Autodesk Inventor part; units mm, degrees
ref_plane "YZ Plane" through (0, 0, 0) normal (1, 0, 0) x (0, 1, 0)
ref_plane "XZ Plane" through (0, 0, 0) normal (0, 1, 0) x (-1, 0, 0)
ref_plane "XY Plane" through (0, 0, 0) normal (0, 0, 1) x (1, 0, 0)
sketch "Sketch1" plane through (0, 0, 0) normal (0, 0, 1) x (1, 0, 0)
  line L0 (-15.7, 12.7) -> (-12.7, 12.7)
  line L1 (-12.7, 12.7) -> (-12.7, -9.7)
  line L2 (-12.7, -9.7) -> (12.7, -9.7)
  line L3 (12.7, -9.7) -> (12.7, 12.7)
  line L4 (12.7, 12.7) -> (15.7, 12.7)
  line L5 (15.7, 12.7) -> (15.7, -12.7)
  line L6 (15.7, -12.7) -> (-15.7, -12.7)
  line L7 (-15.7, -12.7) -> (-15.7, 12.7)
  point P0 (0, 0)
  dimension "d0" = 3
  dimension "d2" = 3
  dimension "d3" = 25.4
  dimension "d4" = 31.4
  dimension "d5" = 15.7
  dimension "d7" = 12.7
  dimension "d8" = 3
extrude "Extrusion1" add sketch "Sketch1" against normal blind 660.4
sketch "Sketch5" plane through (15.7, -12.7, 0) normal (1, 0, 0) x (0, 0, -1)
  circle A0 centre (16, 12.7) radius 3.175
  circle A1 centre (644.4, 12.7) radius 3.175
  line L0 (0, 25.4) -> (0, 0)
  line L1 (660.4, 25.4) -> (660.4, 0)
  line L2 (0, 25.4) -> (660.4, 25.4)
  point P0 (0, 12.7)
  dimension "d56" = 6.35
  dimension "d65" = 6.35
  dimension "d70" = 16
  dimension "d71" = 25.4
  dimension "d72" = 12.7
  dimension "d73" = 16
extrude "Extrusion5" cut sketch "Sketch5" against normal blind 76.2
sketch "Sketch6" plane through (-15.7, -12.7, 0) normal (-1, 0, 0) x (0, 0, 1)
  circle A0 centre (-37.4708, 12.3) radius 3.175
  circle A1 centre (-177.8, 12.3) radius 3.175
  circle A2 centre (-340.3166, 12.3) radius 3.175
  point P0 (0, 12.7)
extrude "Extrusion6" cut sketch "Sketch6" against normal blind 50.8
equation "\"d2\" = d0"
equation "\"d8\" = d0"
equation "\"d65\" = d64"
equation "\"d72\" = 0.5 * d71"
equation "\"d73\" = d70"
equation "\"d58\" = d56"
equation "\"d59\" = d58"
equation "\"d60\" = d59"
equation "\"d61\" = d60"
equation "\"d62\" = d61"
equation "\"d63\" = d62"
equation "\"d64\" = d63"
properties part number "26in C-Channel Right" material "Aluminum 6061"
The model under review builds one solid part; all positions refer to its coordinate system, in mm. A direction names the side the tool comes from. Coordinates: 2 decimals unless noted, no trailing zeros. Write each loop counter-clockwise with the first axis right and the second up, starting at its lowest first coordinate (ties: lowest second). Pieces come first, ordered by that corner, then holes. Notation, with made-up numbers: (76, -3) - (85, -3) arc R10 cw to (85, 7) - close; hole circle Ø7 at (33, -16). An arc over 180 degrees is marked (long way). Answer in a Markdown table with one row per item. Add a question column.
Q1. For faces 5 (the face through (12.7, 1, -326)), 6 (the face through (15.7, 0, -326)), list the 3-axis set-ups (+Z, -Z, +X, -X, +Y, -Y) from which the entire face can be reached by the end or side of a thin tool; tool diameter is ignored.
Q2. Consider section B-B on z = -479.5. Give the boundary of the cut face in (x, y).
Q3. To check wall thickness, follow line 1 along X through (y, z) = (-5.5, -207); line 2 along Y through (x, z) = (-13.85, -177.8) (3 decimals); line 3 along Y through (x, z) = (8, -369). State the ranges of each line that lie inside material, in increasing order. Write a range as from..to.
Q4. Clearance check with flat-ended pins moving along their axes: pin 1 (12 mm diameter, centred on x = 11, z = -385.5, fed in from +Y); pin 2 (5 mm diameter, centred on x = -1, z = -251.5, fed in from +Y). State where each tip first meets the part, or that it passes through.
Q5. Draft analysis for pull direction X (two halves, no side actions). For faces 1 (the face through (-12.7, 2, -326)), 2 (the face through (-15.7, 0, -326)), 3 (the face through (0, -9.7, -326)), 4 (the face through (0, -12.7, -326)), state which applies: +X half, -X half, draft (parallel to the pull), parting line (faces both ways), or undercut.
Q6. Consider section A-A on y = 8.75. Give the boundary of the cut face in (x, z).
Q7. Consider section C-C on x = -5.5. Give the boundary of the cut face in (y, z).
Answers below:
| question | item | result |
|---|---|---|
| 1 | face 5 | +Z, -Z, +Y |
| 1 | face 6 | +Z, -Z, +X, +Y, -Y |
| 2 | outline | (-15.7, -12.7) - (15.7, -12.7) - (15.7, 12.7) - (12.7, 12.7) - (12.7, -9.7) - (-12.7, -9.7) - (-12.7, 12.7) - (-15.7, 12.7) - close |
| 3 | line 1 | -15.7..-12.7, 12.7..15.7 |
| 3 | line 2 | -12.7..-3.575, 2.775..12.7 |
| 3 | line 3 | -12.7..-9.7 |
| 4 | pin 1 | y = 12.7 |
| 4 | pin 2 | y = -9.7 |
| 5 | face 1 | undercut |
| 5 | face 2 | -X half |
| 5 | face 3 | undercut |
| 5 | face 4 | draft |
| 6 | outline | (-15.7, -660.4) - (-12.7, -660.4) - (-12.7, 0) - (-15.7, 0) - close; (12.7, -660.4) - (15.7, -660.4) - (15.7, 0) - (12.7, 0) - close |
| 7 | outline | (-12.7, -660.4) - (-9.7, -660.4) - (-9.7, 0) - (-12.7, 0) - close |
